```python
from build123d import *

# Parameters (mm, degrees)
F1_DEPTH = 12.7
F3_R     = 6.35
F4_DEPTH = 25.4
F2_R     = 4.445
F5_DEPTH = 25.4
F6_W     = 8.89
F6_H     = 25.4
F7_DEPTH = 6.35


with BuildPart() as f1:
    # F0 (on Top) → F1 (new body)
    with BuildSketch(Plane.XY):
        Polygon((152.4, -114.3), (152.4, 114.3), (50.8, 114.3), (50.8, -25.4), (-50.8, -25.4), (-50.8, 114.3), (-152.4, 114.3), (-152.4, -114.3), align=None)
    extrude(amount=F1_DEPTH)

    # F3 (on face) → F4 (cut)
    with BuildSketch(Plane.XY.offset(12.7)):
        with Locations((-88.9, 0)):
            Circle(F3_R)
    extrude(amount=-F4_DEPTH, mode=Mode.SUBTRACT)

    # F2 (on face) → F5 (cut)
    with BuildSketch(Plane.XY.offset(12.7)):
        with Locations((-88.9, 105.41)):
            Circle(F2_R)
        with Locations((88.9, 105.41)):
            Circle(F2_R)
    extrude(amount=-F5_DEPTH, mode=Mode.SUBTRACT)

    # F6 (on face) → F7 (join)
    with BuildSketch(Plane(origin=(0, 0, 0), x_dir=(1, 0, 0), z_dir=(0, 0, -1))):
        Polygon((83.7010406738, -39.3148613891), (77.4148613891, -45.6010406738), (95.3753736312, -63.561552916), (101.661552916, -57.2753736312), align=None)
        with Locations((0, 50.8)):
            Rectangle(F6_W, F6_H)
        Polygon((-95.3753736312, -63.561552916), (-77.4148613891, -45.6010406738), (-83.7010406738, -39.3148613891), (-101.661552916, -57.2753736312), align=None)
    extrude(amount=F7_DEPTH)


solid = f1.part
```
For this review, take the finished solid that the model builds, in its own axes (mm). A direction names the side the tool comes from. Round coordinates to 2 decimals unless told otherwise and drop trailing zeros. Loops run counter-clockwise (first coordinate to the right, second up) from the corner with the lowest first, then second, coordinate; pieces in that order, holes last.
(1) We need section D-D (y = 0). Give the boundary of the cut face in (x, z), plus the area to 3 significant figures.
Returned:
outline: (-152.4, 0) - (-95.25, 0) - (-95.25, 12.7) - (-152.4, 12.7) - close; (-82.55, 0) - (-50.8, 0) - (-50.8, 12.7) - (-82.55, 12.7) - close; (50.8, 0) - (152.4, 0) - (152.4, 12.7) - (50.8, 12.7) - close
area: 2,420 mm2
(2) Clearance check with flat-ended pins moving along their axes: P1, Ø1.9, axis at x = 2, z = -4.5, coming from the -Y side; P2, Ø5, axis at y = -46, z = -4.5, coming from the +X side (3 decimals); P3, Ø1.5, axis at x = 4, z = 4.5, coming from the +Y side. State where each tip first meets the part, or that it passes through.
Returned:
P1: stops at y = -63.5
P2: stops at x = 4.445
P3: stops at y = -25.4
(3) Wall thickness on line 1 along Y through (x, z) = (-88.9, 6) (3 decimals); line 2 along X through (y, z) = (-15.5, 7.5); line 3 along Z through (x, y) = (62.5, 18.5): over which ranges is each line inside the solid? List them lowest first.
Returned:
line 1: y = -114.3 to -6.35, 6.35 to 100.965, 109.855 to 114.3
line 2: x = -152.4 to -50.8, 50.8 to 152.4
line 3: z = 0 to 12.7
(4) We need section B-B (x = 88.9). Give the boundary of the cut face in (y, z) (3 decimals), plus the area to 3 significant figures.
Returned:
outline: (-114.3, 0) - (44.514, 0) - (44.514, -6.35) - (57.086, -6.35) - (57.086, 0) - (100.965, 0) - (100.965, 12.7) - (-114.3, 12.7) - close; (109.855, 0) - (114.3, 0) - (114.3, 12.7) - (109.855, 12.7) - close
area: 2,870 mm2
(5) Tool access review of faces 4 (the flat face through (1, -25.4, 6)), 5 (the flat face through (86.269, 54.456, -3.131)), 6 (the flat face through (98.474, 60.462, -3.131)), 7 (the flat face through (80.602, 42.414, -3.131)), 8 (the flat face through (-101, 114.3, 6)): name each direction out of +Z, -Z, +X, -X, +Y, -Y from which nothing blocks a thin tool from reaching the whole face with its end or side.
Returned:
face 4: +Z, -Z, +Y
face 5: -Z, +Y
face 6: -Z, +X, +Y
face 7: -Z, -Y
face 8: +Z, -Z, +X, -X, +Y
(6) Mouldability with a two-part tool opening along Y and no side actions: class faces 1 (the flat face through (4.445, -51, -3)), 2 (the cylindrical face through (-82.843, 1.907, 6.439)), 3 (the flat face through (-98.562, 60.374, -3.131)) as released by +Y, released by -Y, zero draft, split by the parting line, or undercut.
Returned:
face 1: zero draft
face 2: undercut
face 3: released by +Y
(7) We need section A-A (y = 97). Give the boundary of the cut face in (x, z).
Returned:
outline: (-152.4, 0) - (-50.8, 0) - (-50.8, 12.7) - (-152.4, 12.7) - close; (50.8, 0) - (152.4, 0) - (152.4, 12.7) - (50.8, 12.7) - close
(8) We need section C-C (z = 8). Give the boundary of the cut face in (x, y) (3 decimals).
Returned:
outline: (-152.4, -114.3) - (152.4, -114.3) - (152.4, 114.3) - (50.8, 114.3) - (50.8, -25.4) - (-50.8, -25.4) - (-50.8, 114.3) - (-152.4, 114.3) - close; hole circle Ø12.7 at (-88.9, 0); hole circle Ø8.89 at (-88.9, 105.41); hole circle Ø8.89 at (88.9, 105.41)
